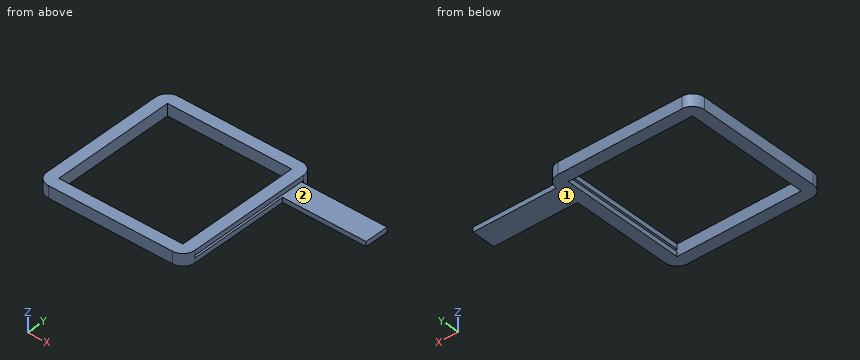
from build123d import *

# Parameters (mm, degrees)
F0_W     = 52
F0_H     = 52
F1_DEPTH = 5
F0_W_2   = 35
F0_H_2   = 10
F2_DEPTH = 2
F4_DEPTH = 5


with BuildPart() as f1:
    # F0 (on Top) → F1 (new body)
    with BuildSketch(Plane.XY):
        with BuildLine():
            Line((57, 0), (5, 0))
            ThreePointArc((5, 0), (1.464466, -1.464466), (0, -5))
            Line((0, -5), (0, -57))
            ThreePointArc((0, -57), (1.464466, -60.535534), (5, -62))
            Line((5, -62), (57, -62))
            ThreePointArc((57, -62), (60.535534, -60.535534), (62, -57))
            Line((62, -57), (62, -15))
            Line((62, -15), (62, -5))
            ThreePointArc((62, -5), (60.535534, -1.464466), (57, 0))
        make_face()
        with Locations((31, -31)):
            Rectangle(F0_W, F0_H, mode=Mode.SUBTRACT)
    extrude(amount=F1_DEPTH)

    # F0 (on Top) → F2 (join)
    with BuildSketch(Plane.XY):
        with Locations((79.5, -10)):
            Rectangle(F0_W_2, F0_H_2)
    extrude(amount=F2_DEPTH)

    # F3 (on face) → F4 (cut, through all)
    with BuildSketch(Plane.YZ.offset(62)):
        Polygon((-15, 2), (-5, 2), (-5, 3), (-57, 3), (-57, 2), align=None)
    extrude(amount=-F4_DEPTH, mode=Mode.SUBTRACT)


solid = f1.part
For this review, take the finished solid that the model builds, in its own axes (mm). Face numbers are marked on the shaded views. Give positions to 0.01 mm unless a question says otherwise; leave off trailing zeros. Loops run counter-clockwise (first coordinate to the right, second up) from the corner with the lowest first, then second, coordinate; pieces in that order, holes last. Notation, with made-up numbers: (11, -18) -> (18, -18) arc R15 cw to (18, 6) -> close; hole circle Ø6 at (-20, 71.25). An arc over 180 degrees is marked (long way). One line per question, with ' | ' between items.
1) We need section D-D (y = -3.5). Write out the cut boundary in (x, z).
Resolved:
outline: (0.23, 0) -> (61.77, 0) -> (61.77, 5) -> (0.23, 5) -> close
2) We need section A-A (x = 31). Write out the cut boundary in (y, z).
Resolved:
outline: (-62, 0) -> (-57, 0) -> (-57, 5) -> (-62, 5) -> close; (-5, 0) -> (0, 0) -> (0, 5) -> (-5, 5) -> close
3) To check wall thickness, follow probe 1 along Y at (x, z) = (15, 1.65); probe 2 along X at (y, z) = (-37.5, 0.9); probe 3 along X at (y, z) = (-11, 1). State the ranges of each line that lie inside material, in increasing order.
Resolved:
probe 1: y = -62 to -57, -5 to 0 | probe 2: x = 0 to 5, 57 to 62 | probe 3: x = 0 to 5, 57 to 97
4) We need section B-B (y = -50). Write out the cut boundary in (x, z).
Resolved:
outline: (0, 0) -> (5, 0) -> (5, 5) -> (0, 5) -> close; (57, 0) -> (62, 0) -> (62, 2) -> (57, 2) -> close; (57, 3) -> (62, 3) -> (62, 5) -> (57, 5) -> close
5) We need section C-C (x = 83). Write out the cut boundary in (y, z), plus the area to 3 significant figures.
Resolved:
outline: (-15, 0) -> (-5, 0) -> (-5, 2) -> (-15, 2) -> close | area: 20.0 mm2
6) The part is to be moulded in two halves that separate along Y. For the marked faces 1 and 2, say which applies: +Y half, -Y half, draft (parallel to the pull), parting line (faces both ways), or undercut.
Resolved:
face 1: draft | face 2: undercut
7) Insertion check: pin 1 Ø1.6 at (x, z) = (77, 1) entering from +Y; pin 2 Ø0.6 at (y, z) = (-35, 0.5) entering from +X; pin 3 Ø0.6 at (x, z) = (83.5, 1.5) entering from -Y. Each pin has a flat end and moves straight along its axis. Give the tip position at first contact, or say it passes through.
Resolved:
pin 1: stops at y = -5 | pin 2: stops at x = 62 | pin 3: stops at y = -15
